The listing builds one solid part. Answer for the finished solid, in the listing's coordinates (mm). A direction names the side the tool comes from. Give positions to 0.01 mm unless a question says otherwise; leave off trailing zeros. Write each loop counter-clockwise with the first axis right and the second up, starting at its lowest first coordinate (ties: lowest second). Pieces come first, ordered by that corner, then holes. Notation, with made-up numbers: (-13, 71) - (41, 71) arc R15 cw to (41, 96) - close; hole circle Ø3 at (44, -31.5). An arc over 180 degrees is marked (long way). One line per question, with ' | ' between items. Start each with the question number.
1. Given P1, Ø0.9, axis at y = 2, z = -6.5, coming from the -X side; P2, Ø0.6, axis at x = 0, y = 1.5, coming from the -Z side; P3, Ø0.6, axis at x = 39.5, y = 1.5, coming from the +Z side, each flat-ended and moving along its own axis, determine where each tip first touches the part or whether it passes through.
2. A cutting plane is placed at B-B (y = 6). Determine the outline of the cut face in (x, z).
3. A cutting plane is placed at D-D (y = 0.75). Determine the outline of the cut face in (x, z), then the cut area to 3 significant figures.
4. The mould has two halves that part along Z. Classify faces 1 (the face through (19.72, 8.34, 19.88)), 2 (the face through (40, 2, 0)), 3 (the face through (19.72, 1.97, -18.21)): +Z half, -Z half, draft (parallel to the pull), parting line (faces both ways), or undercut.
5. A cutting plane is placed at A-A (x = 24). Determine the outline of the cut face in (y, z), then the cut area to 3 significant figures.
6. For faces 4 (the face through (20.28, 3.413, 12.591)), 5 (the face through (0.5, 2, 7)), 6 (the face through (39.5, 2, -6)), determine the directions among +Z, -Z, +X, -X, +Y, -Y from which every point of the face is accessible in a straight line to the end or side of a thin tool.
7. Find the intervals of material crossed by L1, parallel to Z at x = 30, y = 6.25; L2, parallel to Z at x = 31, y = 7.25; L3, parallel to Y at x = 33.5, z = 3.5, in increasing order. Write a range as from..to.
8. A cutting plane is placed at C-C (z = -17). Determine the outline of the cut face in (x, y), then the cut area to 3 significant figures.
```python
from build123d import *

# Parameters (mm, degrees)
SKETCH_1_R          = 1.5
EXTRUDE_1_DEPTH     = 40
FILLET_1_R          = 3
SKETCH_2_W          = 0.5
SKETCH_2_H          = 3
CUT_EXTRUDE_1_DEPTH = 46.57411546


with BuildPart() as part:
    # 스케치1 → 보스-돌출1 (new body)
    with BuildSketch(Plane(origin=(0, 0, 0), x_dir=(0, 0, -1), z_dir=(1, 0, 0))):
        with BuildLine():
            Line((-15.401923789, 7.5), (-12.803847577, 3))
            Line((-12.803847577, 3), (12.803847577, 3))
            Line((12.803847577, 3), (15.401923789, 7.5))
            ThreePointArc((15.401923789, 7.5), (19.826284287, 8.380060021), (20.121320344, 3.878679656))
            Line((20.121320344, 3.878679656), (16.242640687, 0))
            Line((16.242640687, 0), (0, 0))
            Line((0, 0), (-16.242640687, 0))
            Line((-16.242640687, 0), (-20.121320344, 3.878679656))
            ThreePointArc((-20.121320344, 3.878679656), (-19.826284287, 8.380060021), (-15.401923789, 7.5))
        make_face()
        with Locations((18, 6)):
            Circle(SKETCH_1_R, mode=Mode.SUBTRACT)
        with Locations(Location((-18, 6, 0), (0, 0, 180))):
            Circle(SKETCH_1_R, mode=Mode.SUBTRACT)
    extrude(amount=EXTRUDE_1_DEPTH)

    # 필렛1
    fillet_1_edges = [part.edges().sort_by_distance(p)[0] for p in [
        (20, 3, 12.803847577),
        (20, 3, -12.803847577),
    ]]
    fillet(fillet_1_edges, radius=FILLET_1_R)

    # 스케치2 → 컷-돌출1 (cut, through all)
    with BuildSketch(Plane(origin=(0, 3, 0), x_dir=(1, 0, 0), z_dir=(0, 1, 0))):
        with Locations((0.25, 6.5)):
            Rectangle(SKETCH_2_W, SKETCH_2_H)
        with Locations((0.25, -6.5)):
            Rectangle(SKETCH_2_W, SKETCH_2_H)
        with Locations((39.75, 6.5)):
            Rectangle(SKETCH_2_W, SKETCH_2_H)
        with Locations((39.75, -6.5)):
            Rectangle(SKETCH_2_W, SKETCH_2_H)
    extrude(amount=-CUT_EXTRUDE_1_DEPTH, mode=Mode.SUBTRACT)


solid = part.part
```
Determined:
1) P1: x = 0.5 | P2: z = -18.04 | P3: z = 18.04
2) outline: (0, -21) - (40, -21) - (40, -19.5) - (0, -19.5) - close; (0, -16.5) - (40, -16.5) - (40, -14.54) - (0, -14.54) - close; (0, 14.54) - (40, 14.54) - (40, 16.5) - (0, 16.5) - close; (0, 19.5) - (40, 19.5) - (40, 21) - (0, 21) - close
3) outline: (0, -16.99) - (40, -16.99) - (40, -8) - (39.5, -8) - (39.5, -5) - (40, -5) - (40, 5) - (39.5, 5) - (39.5, 8) - (40, 8) - (40, 16.99) - (0, 16.99) - (0, 8) - (0.5, 8) - (0.5, 5) - (0, 5) - (0, -5) - (0.5, -5) - (0.5, -8) - (0, -8) - close | area: 1,350 mm2
4) face 1: undercut | face 2: draft | face 3: -Z half
5) outline: (0, -16.24) - (3.88, -20.12) arc R3 ccw (long way) to (7.5, -15.4) - (4.5, -13.67) arc R3 cw to (3, -11.07) - (3, 11.07) arc R3 cw to (4.5, 13.67) - (7.5, 15.4) arc R3 ccw (long way) to (3.88, 20.12) - (0, 16.24) - close; hole circle Ø3 at (6, -18); hole circle Ø3 at (6, 18) | area: 163 mm2
6) face 4: +X, -X, +Y | face 5: -X, +Y, -Y | face 6: +X, +Y, -Y
7) L1: -20.99..-19.48, -16.52..-14.68, 14.68..16.52, 19.48..20.99 | L2: -20.73..-18.83, -17.17..-15.26, 15.26..17.17, 18.83..20.73 | L3: 0..3
8) outline: (0, 0.76) - (40, 0.76) - (40, 4.88) - (0, 4.88) - close; (0, 7.12) - (40, 7.12) - (40, 8.83) - (0, 8.83) - close | area: 233 mm2
